The listing builds one solid part. Answer for the finished solid, in the listing's coordinates (mm). Coordinates: 2 decimals unless noted, no trailing zeros. Loops run counter-clockwise (first coordinate to the right, second up) from the corner with the lowest first, then second, coordinate; pieces in that order, holes last. Notation, with made-up numbers: M 31,54.25 L 59,54.25 A26 cw 59,78.25 Z; hole C 37.5,69.25 d6. An arc over 180 degrees is marked long. Answer as a JSON object with one key per item and string values. Group by question number.
1. A cutting plane is placed at A-A on z = 8.75. Give the vertices of the cut face in (x, y), and give its area (3 significant figures).
2. Determine the mould class of faces 1 (the face through (-10.008, 0.789, -11.274)), 2 (the face through (-20, 1, 0)), 3 (the face through (0, 1, 13.75)) for opening direction Z: released by +Z, released by -Z, zero draft, split by the parting line, or undercut.
3. A cutting plane is placed at B-B on x = -9.5. Give the vertices of the cut face in (y, z).
4. A cutting plane is placed at C-C on y = 0.5. Give the vertices of the cut face in (x, z).
5. Straight lines are drawn through the part: L1, parallel to Z at x = -9.5, y = 1.3; L2, parallel to X at y = 1.1, z = 8.75; L3, parallel to X at y = 0.5, z = -12.25. For each, find the intervals that lie inside material, in ascending order.
from build123d import *

# Parameters (mm, degrees)
SKETCH1_W                = 40
SKETCH1_H                = 27.5
BOSS_EXTRUDE1_DEPTH      = 1.6
M2_CLEARANCE_HOLE1_D     = 2.2
M2_CLEARANCE_HOLE1_DEPTH = 5.2
M2_CLEARANCE_HOLE1_TIP   = 0.660946681
FILLET1_R                = 3


with BuildPart() as part:
    # Sketch1 → Boss-Extrude1 (new body)
    with BuildSketch(Plane(origin=(0, 0, 0), x_dir=(1, 0, 0), z_dir=(0, 1, 0))):
        Rectangle(SKETCH1_W, SKETCH1_H)
    extrude(amount=BOSS_EXTRUDE1_DEPTH)

    # M2 Clearance Hole1
    with Locations(Plane(origin=(0, 1.6, 0), x_dir=(1, 0, 0), z_dir=(0, 1, 0))):
        with Locations((-9.5, 12.25), (9.5, 12.25), (9.5, -8.75), (-9.5, -8.75)):
            Hole(M2_CLEARANCE_HOLE1_D / 2, depth=M2_CLEARANCE_HOLE1_DEPTH)
            with Locations((0, 0, -(M2_CLEARANCE_HOLE1_DEPTH + M2_CLEARANCE_HOLE1_TIP / 2))):  # 118° drill point
                Cone(0, M2_CLEARANCE_HOLE1_D / 2, M2_CLEARANCE_HOLE1_TIP, mode=Mode.SUBTRACT)

    # Fillet1
    fillet1_edges = [part.edges().sort_by_distance(p)[0] for p in [
        (-20, 0.8, -13.75),
        (20, 0.8, -13.75),
        (20, 0.8, 13.75),
        (-20, 0.8, 13.75),
    ]]
    fillet(fillet1_edges, radius=FILLET1_R)


solid = part.part
From the geometry:
{
 "1": {"outline": "M -20,0 L -10.6,0 L -10.6,1.6 L -20,1.6 Z; M -8.4,0 L 8.4,0 L 8.4,1.6 L -8.4,1.6 Z; M 10.6,0 L 20,0 L 20,1.6 L 10.6,1.6 Z", "area": "57.0 mm²"},
 "2": {"face 1": "undercut", "face 2": "zero draft", "face 3": "released by +Z"},
 "3": {"outline": "M 0,-13.75 L 1.6,-13.75 L 1.6,-13.35 L 0,-13.35 Z; M 0,-11.15 L 1.6,-11.15 L 1.6,7.65 L 0,7.65 Z; M 0,9.85 L 1.6,9.85 L 1.6,13.75 L 0,13.75 Z"},
 "4": {"outline": "M -20,-10.75 A3 ccw -17,-13.75 L 17,-13.75 A3 ccw 20,-10.75 L 20,10.75 A3 ccw 17,13.75 L -17,13.75 A3 ccw -20,10.75 Z; hole C -9.5,-12.25 d2.2; hole C -9.5,8.75 d2.2; hole C 9.5,-12.25 d2.2; hole C 9.5,8.75 d2.2"},
 "5": {"L1": "z = -13.75 to -13.35, -11.15 to 7.65, 9.85 to 13.75", "L2": "x = -20 to -10.6, -8.4 to 8.4, 10.6 to 20", "L3": "x = -19.6 to -10.6, -8.4 to 8.4, 10.6 to 19.6"}
}
